The listing builds one solid part. Answer for the finished solid, in the listing's coordinates (mm). Face numbers are marked on the shaded views. Give positions to 0.01 mm unless a question says otherwise; leave off trailing zeros. Order: outer loops, then holes, each group sorted by start corner. A loop starts at its lowest first (then second) coordinate and runs counter-clockwise, first axis right, second up. Notation, with made-up numbers: (-10, 76.5) - (46, 76.5) arc R26 cw to (46, 90.5) - close; hole circle Ø11 at (68, 10). An arc over 180 degrees is marked (long way). Use CSV: the item, a comma, the result in double quotes.
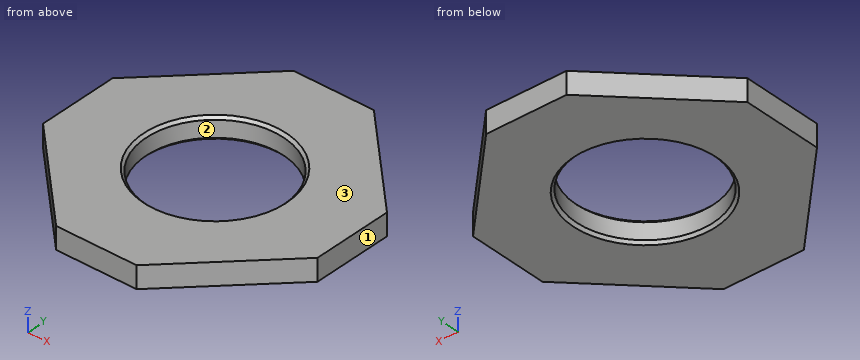
Autodesk Inventor part; units mm, degrees
ref_plane "YZ Plane" through (0, 0, 0) normal (1, 0, 0) x (0, 1, 0)
ref_plane "XZ Plane" through (0, 0, 0) normal (0, 1, 0) x (-1, 0, 0)
ref_plane "XY Plane" through (0, 0, 0) normal (0, 0, 1) x (1, 0, 0)
sketch "Esquisse1" plane through (0, 0, 0) normal (0, 0, 1) x (1, 0, 0)
  circle A0 centre (0, 0) radius 25
  line L0 (-50, 14.6447) -> (-14.6447, 50)
  line L1 (14.6447, 50) -> (50, 14.6447)
  line L2 (50, -14.6447) -> (14.6447, -50)
  line L3 (-14.6447, -50) -> (-50, -14.6447)
  line L4 (-70, 0) -> (70, 0) construction
  line L5 (0, -70) -> (0, 70) construction
  line L6 (50, -14.6447) -> (50, 14.6447)
  line L7 (-50, -14.6447) -> (-50, 14.6447)
  line L8 (-14.6447, 50) -> (14.6447, 50)
  line L9 (-14.6447, -50) -> (14.6447, -50)
  dimension "d0" = 50
  dimension "d9" = 100
  dimension "d11" = 45
  dimension "d12" = 50
  dimension "d13" = 100
  dimension "d14" = 50
  dimension "d15" = 50
extrude "Extrusion1" add sketch "Esquisse1" along normal blind 8
chamfer "Chanfrein1" distance 1 angle 45 2 edges at (-25, 0, 8) (-25, 0, 0)
equation "\"d13\" = d9"
equation "\"d14\" = 0.5 * d13"
properties part number "support_bois_reservoir"
Item 1: The part is cut by section A-A (x = 0). Give the vertices of the cut face in (y, z), and give its area (3 significant figures).
Taken from the geometry:
outline,"(-50, 0) - (-26, 0) - (-25, 1) - (-25, 7) - (-26, 8) - (-50, 8) - close; (25, 1) - (26, 0) - (50, 0) - (50, 8) - (26, 8) - (25, 7) - close"
area,"398 mm^2"
Item 2: The part is cut by section C-C (z = 3). Give the vertices of the cut face in (x, y), and give its area (3 significant figures).
Taken from the geometry:
outline,"(-50, -14.64) - (-14.64, -50) - (14.64, -50) - (50, -14.64) - (50, 14.64) - (14.64, 50) - (-14.64, 50) - (-50, 14.64) - close; hole circle Ø50 at (0, 0)"
area,"5,540 mm^2"
Item 3: Find the intervals of material crossed by line 1 along Y through (x, z) = (0, 5.35); line 2 along Y through (x, z) = (-21, 5.25); line 3 along X through (y, z) = (-13, 1.5), in increasing order.
Taken from the geometry:
line 1,"-50 to -25, 25 to 50"
line 2,"-43.64 to -13.56, 13.56 to 43.64"
line 3,"-50 to -21.35, 21.35 to 50"
Item 4: Each of these flat-tipped pins is pushed along its axis until it touches: pin 1 (1 mm diameter, centred on y = -30.5, z = 2.5, fed in from +X); pin 2 (2 mm diameter, centred on y = -40, z = 2, fed in from -X); pin 3 (2 mm diameter, centred on y = -36, z = 6.5, fed in from -X). Where does it stop, or does it pass through?
Taken from the geometry:
pin 1,"x = 34.64"
pin 2,"x = -25.64"
pin 3,"x = -29.64"
Item 5: The mould has two halves that part along X. Classify the marked faces 1, 2 and 3: +X half, -X half, draft (parallel to the pull), parting line (faces both ways), or undercut.
Taken from the geometry:
face 1,"+X half"
face 2,"undercut"
face 3,"draft"
Item 6: The part is cut by section D-D (x = 29.5). Give the vertices of the cut face in (y, z), and give its area (3 significant figures).
Taken from the geometry:
outline,"(-35.14, 0) - (35.14, 0) - (35.14, 8) - (-35.14, 8) - close"
area,"562 mm^2"
